Verification items for the finished model (mm, model axes). A direction names the side the tool comes from. Round coordinates to 2 decimals unless told otherwise and drop trailing zeros. Order: outer loops, then holes, each group sorted by start corner. A loop starts at its lowest first (then second) coordinate and runs counter-clockwise, first axis right, second up. Notation, with made-up numbers: (74, 15) -> (93, 15) arc R15 cw to (93, 43) -> close; hole circle Ø6 at (-34, 87.5). An arc over 180 degrees is marked (long way). Put each result on its own line as item: value.
```python
from build123d import *
from OCP.BRepFilletAPI import BRepFilletAPI_MakeChamfer

# Parameters (mm, degrees)
SALIENTE_EXTRUIR1_DEPTH = 2
SALIENTE_EXTRUIR2_DEPTH = 2
CORTAR_EXTRUIR1_DEPTH   = 2
CROQUIS5_R              = 28.015207884
CROQUIS5_R_2            = 27.015207884
CROQUIS5_R_3            = 3
CORTAR_EXTRUIR2_DEPTH   = 0.8
CROQUIS6_R              = 2.7
CORTAR_EXTRUIR3_DEPTH   = 11.8
CROQUIS7_R              = 3
SALIENTE_EXTRUIR3_DEPTH = 31.34
CROQUIS8_R              = 2
CORTAR_EXTRUIR4_DEPTH   = 5
CROQUIS9_W              = 20.569885585
CROQUIS9_H              = 2.86791674
CORTAR_EXTRUIR5_DEPTH   = 1
CROQUIS10_W             = 0.685574001
CROQUIS10_H             = 8.330017526
CROQUIS10_W_2           = 0.70136351
SALIENTE_EXTRUIR4_DEPTH = 1
CROQUIS11_W             = 1.000377771
CROQUIS11_H             = 8.330017526
SALIENTE_EXTRUIR5_DEPTH = 0.3
CROQUIS12_W             = 1.006924042
CROQUIS12_H             = 8.323274802
SALIENTE_EXTRUIR6_DEPTH = 0.5
CHAFL_N1_SIZE           = 0.310659094
CHAFL_N1_SIZE_2         = 0.3
CORTAR_EXTRUIR6_DEPTH   = 0.8


with BuildPart() as part:
    # Croquis1 → Saliente-Extruir1 (new body)
    with BuildSketch(Plane.XY):
        with BuildLine():
            Line((-24.066972173, 40), (-24.066972173, -40))
            ThreePointArc((-24.066972173, -40), (-21.181973968, -46.965001795), (-14.216972173, -49.85))
            Line((-14.216972173, -49.85), (65.783027827, -49.85))
            ThreePointArc((65.783027827, -49.85), (72.748029622, -46.965001795), (75.633027827, -40))
            Line((75.633027827, -40), (75.633027827, 40))
            ThreePointArc((75.633027827, 40), (72.748029622, 46.965001795), (65.783027827, 49.85))
            Line((65.783027827, 49.85), (-14.216972173, 49.85))
            ThreePointArc((-14.216972173, 49.85), (-21.181973968, 46.965001795), (-24.066972173, 40))
        make_face()
    extrude(amount=SALIENTE_EXTRUIR1_DEPTH)

    # Croquis2 → Saliente-Extruir2 (add)
    with BuildSketch(Plane(origin=(0, 0, 0), x_dir=(-1, 0, 0), z_dir=(0, 0, -1))):
        with BuildLine():
            Line((14.216972173, 48.85), (-65.783027827, 48.85))
            ThreePointArc((-65.783027827, 48.85), (-72.040922841, 46.257895014), (-74.633027827, 40))
            Line((-74.633027827, 40), (-74.633027827, -40))
            ThreePointArc((-74.633027827, -40), (-72.040922841, -46.257895014), (-65.783027827, -48.85))
            Line((-65.783027827, -48.85), (14.216972173, -48.85))
            ThreePointArc((14.216972173, -48.85), (20.474867186, -46.257895014), (23.066972173, -40))
            Line((23.066972173, -40), (23.066972173, 40))
            ThreePointArc((23.066972173, 40), (20.474867186, 46.257895014), (14.216972173, 48.85))
        make_face()
    extrude(amount=SALIENTE_EXTRUIR2_DEPTH)

    # Croquis3 → Cortar-Extruir1 (cut)
    with BuildSketch(Plane(origin=(0, 0, -2), x_dir=(-1, 0, 0), z_dir=(0, 0, -1))):
        Polygon((-5.783027827, 0), (-5.783027827, -40), (-45.783027827, -40), (-45.783027827, 0), (-45.783027827, 20.3), (-5.783027827, 20.3), align=None)
    extrude(amount=-CORTAR_EXTRUIR1_DEPTH, mode=Mode.SUBTRACT)

    # Croquis5 → Cortar-Extruir2 (cut)
    # profile 1 of 10: a face of its own
    with BuildSketch(Plane.XY.offset(2)):
        with Locations((25.783027827, 0)):
            Circle(CROQUIS5_R)
        with Locations((25.783027827, 0)):
            Circle(CROQUIS5_R_2, mode=Mode.SUBTRACT)
    # profile 2 of 10: a face of its own
    with BuildSketch(Plane.XY.offset(2)):
        with Locations((25.783027827, 0)):
            Circle(CROQUIS5_R_3)
    # profile 3 of 10: a face of its own
    with BuildSketch(Plane.XY.offset(2)):
        with BuildLine():
            ThreePointArc((40.344100587, -16.491669415), (47.783027827, 0), (40.344100587, 16.491669415))
            ThreePointArc((40.344100587, 16.491669415), (40.30022339, 17.197413555), (41.00596753, 17.241290752))
            ThreePointArc((41.00596753, 17.241290752), (48.783027827, 0), (41.00596753, -17.241290752))
            ThreePointArc((41.00596753, -17.241290752), (40.30022339, -17.197413555), (40.344100587, -16.491669415))
        make_face()
    # profile 4 of 10: a face of its own
    with BuildSketch(Plane.XY.offset(2)):
        with BuildLine():
            ThreePointArc((37.034765869, -12.74356273), (42.783027827, 0), (37.034765869, 12.74356273))
            ThreePointArc((37.034765869, 12.74356273), (36.990888672, 13.44930687), (37.696632812, 13.493184067))
            ThreePointArc((37.696632812, 13.493184067), (43.783027827, 0), (37.696632812, -13.493184067))
            ThreePointArc((37.696632812, -13.493184067), (36.990888672, -13.44930687), (37.034765869, -12.74356273))
        make_face()
    # profile 5 of 10: a face of its own
    with BuildSketch(Plane.XY.offset(2)):
        with BuildLine():
            ThreePointArc((33.725431151, -8.995456045), (37.783027827, 0), (33.725431151, 8.995456045))
            ThreePointArc((33.725431151, 8.995456045), (33.681553954, 9.701200185), (34.387298094, 9.745077382))
            ThreePointArc((34.387298094, 9.745077382), (38.783027827, 0), (34.387298094, -9.745077382))
            ThreePointArc((34.387298094, -9.745077382), (33.681553954, -9.701200185), (33.725431151, -8.995456045))
        make_face()
    # profile 6 of 10: a face of its own
    with BuildSketch(Plane.XY.offset(2)):
        with BuildLine():
            ThreePointArc((30.416096432, -5.247349359), (32.783027827, 0), (30.416096432, 5.247349359))
            ThreePointArc((30.416096432, 5.247349359), (30.372219236, 5.9530935), (31.077963376, 5.996970696))
            ThreePointArc((31.077963376, 5.996970696), (33.783027827, 0), (31.077963376, -5.996970696))
            ThreePointArc((31.077963376, -5.996970696), (30.372219236, -5.9530935), (30.416096432, -5.247349359))
        make_face()
    # profile 7 of 10: a face of its own
    with BuildSketch(Plane.XY.offset(2)):
        with BuildLine():
            ThreePointArc((20.488092278, 5.996970696), (17.783027827, 0), (20.488092278, -5.996970696))
            ThreePointArc((20.488092278, -5.996970696), (21.193836419, -5.9530935), (21.149959222, -5.247349359))
            ThreePointArc((21.149959222, -5.247349359), (18.783027827, 0), (21.149959222, 5.247349359))
            ThreePointArc((21.149959222, 5.247349359), (21.193836419, 5.9530935), (20.488092278, 5.996970696))
        make_face()
    # profile 8 of 10: a face of its own
    with BuildSketch(Plane.XY.offset(2)):
        with BuildLine():
            ThreePointArc((17.17875756, 9.745077382), (12.783027827, 0), (17.17875756, -9.745077382))
            ThreePointArc((17.17875756, -9.745077382), (17.884501701, -9.701200185), (17.840624504, -8.995456045))
            ThreePointArc((17.840624504, -8.995456045), (13.783027827, 0), (17.840624504, 8.995456045))
            ThreePointArc((17.840624504, 8.995456045), (17.884501701, 9.701200185), (17.17875756, 9.745077382))
        make_face()
    # profile 9 of 10: a face of its own
    with BuildSketch(Plane.XY.offset(2)):
        with BuildLine():
            ThreePointArc((13.869422842, 13.493184067), (7.783027827, 0), (13.869422842, -13.493184067))
            ThreePointArc((13.869422842, -13.493184067), (14.575166983, -13.44930687), (14.531289786, -12.74356273))
            ThreePointArc((14.531289786, -12.74356273), (8.783027827, 0), (14.531289786, 12.74356273))
            ThreePointArc((14.531289786, 12.74356273), (14.575166983, 13.44930687), (13.869422842, 13.493184067))
        make_face()
    # profile 10 of 10: a face of its own
    with BuildSketch(Plane.XY.offset(2)):
        with BuildLine():
            ThreePointArc((10.560088124, 17.241290752), (2.783027827, 0), (10.560088124, -17.241290752))
            ThreePointArc((10.560088124, -17.241290752), (11.265832264, -17.197413555), (11.221955068, -16.491669415))
            ThreePointArc((11.221955068, -16.491669415), (3.783027827, 0), (11.221955068, 16.491669415))
            ThreePointArc((11.221955068, 16.491669415), (11.265832264, 17.197413555), (10.560088124, 17.241290752))
        make_face()
    extrude(amount=-CORTAR_EXTRUIR2_DEPTH, mode=Mode.SUBTRACT)

    # Croquis6 → Cortar-Extruir3 (cut)
    with BuildSketch(Plane.XY.offset(2)):
        with Locations((25.783027827, 42.084354259)):
            Circle(CROQUIS6_R)
        with Locations(Location((39.706644574, 42.084354259, 0), (0, 0, 180))):
            Circle(CROQUIS6_R)
        with Locations((11.859411081, 42.084354259)):
            Circle(CROQUIS6_R)
    extrude(amount=-CORTAR_EXTRUIR3_DEPTH, mode=Mode.SUBTRACT)

    # Croquis7 → Saliente-Extruir3 (add)
    with BuildSketch(Plane(origin=(0, 0, -2), x_dir=(-1, 0, 0), z_dir=(0, 0, -1))):
        with Locations(Location((2.62017868, -5.323274802, 0), (0, 0, 180))):
            Circle(CROQUIS7_R)
        with Locations(Location((-59.659023373, 16.754261366, 0), (0, 0, 180))):
            Circle(CROQUIS7_R)
        with Locations(Location((0, 27.466663807, 0), (0, 0, 180))):
            Circle(CROQUIS7_R)
    extrude(amount=SALIENTE_EXTRUIR3_DEPTH)

    # Croquis8 → Cortar-Extruir4 (cut)
    with BuildSketch(Plane(origin=(0, 0, -33.34), x_dir=(-1, 0, 0), z_dir=(0, 0, -1))):
        with Locations((2.62017868, -5.323274802)):
            Circle(CROQUIS8_R)
        with Locations((0, 27.466663807)):
            Circle(CROQUIS8_R)
        with Locations((-59.659023373, 16.754261366)):
            Circle(CROQUIS8_R)
    extrude(amount=-CORTAR_EXTRUIR4_DEPTH, mode=Mode.SUBTRACT)

    # Croquis9 → Cortar-Extruir5 (cut)
    with BuildSketch(Plane(origin=(0, 0, 0), x_dir=(-1, 0, 0), z_dir=(0, 0, -1))):
        with Locations((-25.751233426, -37.742845004)):
            Rectangle(CROQUIS9_W, CROQUIS9_H)
    extrude(amount=-CORTAR_EXTRUIR5_DEPTH, mode=Mode.SUBTRACT)

    # Croquis10 → Saliente-Extruir4 (add)
    with BuildSketch(Plane(origin=(0, 0, -2), x_dir=(-1, 0, 0), z_dir=(0, 0, -1))):
        with Locations((-5.440240827, -4.165008763)):
            Rectangle(CROQUIS10_W, CROQUIS10_H)
        with Locations((-46.133709582, -4.165008763)):
            Rectangle(CROQUIS10_W_2, CROQUIS10_H)
    extrude(amount=SALIENTE_EXTRUIR4_DEPTH)

    # Croquis11 → Saliente-Extruir5 (add)
    with BuildSketch(Plane(origin=(5.783027827, 0, 0), x_dir=(0, 0, -1), z_dir=(1, 0, 0))):
        with Locations((2.499811114, -4.165008763)):
            Rectangle(CROQUIS11_W, CROQUIS11_H)
    extrude(amount=SALIENTE_EXTRUIR5_DEPTH)

    # Croquis12 → Saliente-Extruir6 (add)
    with BuildSketch(Plane.ZY.offset(-45.783027827)):
        with Locations((-2.496537979, -4.161637401)):
            Rectangle(CROQUIS12_W, CROQUIS12_H)
    extrude(amount=SALIENTE_EXTRUIR6_DEPTH)

    # Chaflán1
    chafl_n1_edges_1 = [part.edges().sort_by_distance(p)[0] for p in [
        (45.283027827, -4.161637401, -1.993075958),
    ]]
    chafl_n1_side_1 = [part.faces().sort_by_distance(p)[0] for p in [
        (45.283027827, -4.161637401, -1.999075958),
    ]]
    chafl_n1_edges_2 = [part.edges().sort_by_distance(p)[0] for p in [
        (6.083027827, -4.165008763, -1.999622229),
    ]]
    chafl_n1_side_2 = [part.faces().sort_by_distance(p)[0] for p in [
        (6.077027827, -4.165008763, -1.999622229),
    ]]
    chafl_n1 = BRepFilletAPI_MakeChamfer(part.part.solid().wrapped)
    for e in chafl_n1_edges_1:
        chafl_n1.Add(CHAFL_N1_SIZE - 0.0001, CHAFL_N1_SIZE_2 - 0.0001, e.wrapped, chafl_n1_side_1[0].wrapped)
    for e in chafl_n1_edges_2:
        chafl_n1.Add(CHAFL_N1_SIZE_2 - 0.0001, CHAFL_N1_SIZE - 0.0001, e.wrapped, chafl_n1_side_2[0].wrapped)
    add(Compound.cast(chafl_n1.Shape()), mode=Mode.REPLACE)  # a hair under: the kernel refuses the full size

    # Croquis13 → Cortar-Extruir6 (cut)
    with BuildSketch(Plane.XY.offset(2)):
        with BuildLine():
            ThreePointArc((15.07431414, 37.867927159), (18.821219454, 39.133432517), (22.568124768, 37.867927159))
            ThreePointArc((22.568124768, 37.867927159), (25.783027827, 36.782103872), (28.997930887, 37.867927159))
            ThreePointArc((28.997930887, 37.867927159), (32.7448362, 39.133432517), (36.491741514, 37.867927159))
            ThreePointArc((36.491741514, 37.867927159), (45.008894961, 42.084354259), (36.491741514, 46.300781358))
            ThreePointArc((36.491741514, 46.300781358), (32.7448362, 45.035276001), (28.997930887, 46.300781358))
            ThreePointArc((28.997930887, 46.300781358), (25.783027827, 47.386604646), (22.568124768, 46.300781358))
            ThreePointArc((22.568124768, 46.300781358), (18.821219454, 45.035276001), (15.07431414, 46.300781358))
            ThreePointArc((15.07431414, 46.300781358), (6.557160693, 42.084354259), (15.07431414, 37.867927159))
        make_face()
        with BuildLine():
            ThreePointArc((14.467986105, 45.505566725), (7.557160693, 42.084354259), (14.467986105, 38.663141793))
            ThreePointArc((14.467986105, 38.663141793), (18.821219454, 40.133432517), (23.174452803, 38.663141793))
            ThreePointArc((23.174452803, 38.663141793), (25.783027827, 37.782103872), (28.391602851, 38.663141793))
            ThreePointArc((28.391602851, 38.663141793), (32.7448362, 40.133432517), (37.09806955, 38.663141793))
            ThreePointArc((37.09806955, 38.663141793), (44.008894961, 42.084354259), (37.09806955, 45.505566725))
            ThreePointArc((37.09806955, 45.505566725), (32.7448362, 44.035276001), (28.391602851, 45.505566725))
            ThreePointArc((28.391602851, 45.505566725), (25.783027827, 46.386604646), (23.174452803, 45.505566725))
            ThreePointArc((23.174452803, 45.505566725), (18.821219454, 44.035276001), (14.467986105, 45.505566725))
        make_face(mode=Mode.SUBTRACT)
    extrude(amount=-CORTAR_EXTRUIR6_DEPTH, mode=Mode.SUBTRACT)


solid = part.part
```
Item 1: Sectioned sample at B-B, the plane z = -31. Record the boundary of the cut face in (x, y), then the cut area to 3 significant figures.
Geometry check:
outline: circle Ø6 at (-2.62, -5.32); circle Ø6 at (0, 27.47); circle Ø6 at (59.66, 16.75); hole circle Ø4 at (-2.62, -5.32); hole circle Ø4 at (0, 27.47); hole circle Ø4 at (59.66, 16.75)
area: 47.1 mm2
Item 2: Sectioned sample at C-C, the plane z = -9. Record the boundary of the cut face in (x, y).
Geometry check:
outline: circle Ø6 at (-2.62, -5.32); circle Ø6 at (0, 27.47); circle Ø6 at (59.66, 16.75)
Item 3: Tool access check on faces 1 (the face through (33, 0, 1.2)), 2 (the face through (25, -6, 2)), 3 (the face through (26, -38, 1)). Record the directions out of +Z, -Z, +X, -X, +Y, -Y that give a thin tool (end or side, any length) a straight path to the whole face; none if there is none.
Geometry check:
face 1: +Z
face 2: +Z, +X, -X, +Y, -Y
face 3: -Z
Item 4: Material ranges on line 1 along Z through (x, y) = (35, -37); line 2 along Z through (x, y) = (41.5, -42.5); line 3 along Y through (x, z) = (0, -31.3), recorded low to high.
Geometry check:
line 1: 1 to 2
line 2: -2 to 2
line 3: -6.78 to -3.86, 24.47 to 25.47, 29.47 to 30.47
Item 5: Sectioned sample at A-A, the plane x = -7. Record the boundary of the cut face in (y, z).
Geometry check:
outline: (-49.85, 0) -> (-48.85, 0) -> (-48.85, -2) -> (48.85, -2) -> (48.85, 0) -> (49.85, 0) -> (49.85, 2) -> (-49.85, 2) -> close
Item 6: Depth check by flat-ended pin: pin 1 Ø0.6 at (y, z) = (11, -1) entering from +X; pin 2 Ø2 at (x, z) = (62.5, -19.5) entering from +Y; pin 3 Ø8.5 at (x, y) = (25.78, 42.08) entering from -Z. Enter the tip coordinate at first touch or a pass-through.
Geometry check:
pin 1: x = 74.63
pin 2: y = 19.12
pin 3: z = -2
Item 7: Release check for a two-part mould opening along Y. For faces 4 (the face through (26, 39, 2)), 5 (the face through (72.67, -47.04, 0.99)), 6 (the face through (41.697, 40.26, 0.028)), 7 (the face through (72.82, 46.89, 0.99)) record: pulls with the +Y half, pulls with the -Y half, needs draft (parallel to the pull), parting line crosses it, or undercut.
Geometry check:
face 4: needs draft
face 5: pulls with the -Y half
face 6: undercut
face 7: pulls with the +Y half
